from build123d import *

# Parameters (mm, degrees)
CHANFRO2_SIZE         = 0.3
CORTE_EXTRUS_O2_REACH = 10.374
ESBO_O7_W             = 0.5
ESBO_O7_H             = 0.2
PADR_OCIRCULAR1_COUNT = 8
M2X0_4_TAPPED_HOLE1_D = 1.6


with BuildPart() as part:
    # Esboço2 → Revolução1 (revolve)
    with BuildSketch(Plane.XY, mode=Mode.PRIVATE) as revolu_o1_sk:
        Polygon((0, 8), (1.75, 8), (1.75, 5.7), (1.4, 5.7), (1.4, 2.3), (1.75, 2.3), (1.75, 0), (0, 0), align=None)
    revolve(revolu_o1_sk.sketch.rotate(Axis((0, 0, 0), (0, 1, 0)), 90), axis=Axis((0, 0, 0), (0, 1, 0)))

    # Chanfro2
    chanfro2_edges = [part.edges().sort_by_distance(p)[0] for p in [
        (0, 0, 1.75),
        (0, 8, 1.75),
    ]]
    chamfer(chanfro2_edges, length=CHANFRO2_SIZE)

    # Corte-extrusão2: up to this face of the body (flat: up to its plane)
    corte_extrus_o2_end = Plane(part.part.faces().sort_by_distance((0, 0, 0))[0])
    # Esboço7 → Corte-extrusão2 (cut, up to the picked face)
    with BuildSketch(Plane(origin=(0, 8, 0), x_dir=(1, 0, 0), z_dir=(0, 1, 0)), mode=Mode.PRIVATE) as corte_extrus_o2_sk1:
        with Locations((0, 1.65)):
            Rectangle(ESBO_O7_W, ESBO_O7_H)
    corte_extrus_o2_tool1 = split(extrude(corte_extrus_o2_sk1.sketch, amount=-CORTE_EXTRUS_O2_REACH, mode=Mode.PRIVATE), bisect_by=corte_extrus_o2_end, keep=Keep.BOTH, mode=Mode.PRIVATE)
    corte_extrus_o2 = corte_extrus_o2_tool1.solids().sort_by(Axis((0, 8, -1.65), (0, -1, 0)))[0]
    add(corte_extrus_o2, mode=Mode.SUBTRACT)

    # PadrãoCircular1: Corte-extrusão2 ×8 about axis
    padr_ocircular1_axis = Axis((0, 0, 0), (0, 1, 0))
    for i in range(1, PADR_OCIRCULAR1_COUNT):
        add(corte_extrus_o2.rotate(padr_ocircular1_axis, i * 360 / PADR_OCIRCULAR1_COUNT), mode=Mode.SUBTRACT)

    # M2x0.4 Tapped Hole1 (through all)
    with Locations(Plane(origin=(0, 8, 0), x_dir=(1, 0, 0), z_dir=(0, 1, 0))):
        with Locations((0, 0)):
            Hole(M2X0_4_TAPPED_HOLE1_D / 2)


solid = part.part
Read the model definition and answer for the solid it produces. Units are mm, in the model's axes. Round coordinates to 2 decimals unless told otherwise and drop trailing zeros. Write each loop counter-clockwise with the first axis right and the second up, starting at its lowest first coordinate (ties: lowest second). Pieces come first, ordered by that corner, then holes. Notation, with made-up numbers: (75, 29) - (124, 29) arc R15 ccw to (124, 40) - close; hole circle Ø6 at (36, 54.25). An arc over 180 degrees is marked (long way). One line per question, with ' | ' between items. Start each with the question number.
1. Section A-A (x = 0) is taken. Determine the outline of the cut face in (y, z).
2. Section D-D (y = 2.75) is taken. Determine the outline of the cut face in (x, z).
3. For a pull along Y with two mould halves and no side action, classify faces 1 (the face through (0.63, 3.94, 0.49)), 2 (the face through (-0.06, 3.98, 1.4)), 3 (the face through (0.6, 7.88, -1.45)) as +Y half, -Y half, draft (parallel to the pull), parting line (faces both ways), or undercut.
4. Find the intervals of material crossed by probe 1 along Z at (x, y) = (0.05, 3.25); probe 2 along Z at (x, y) = (0, 2); probe 3 along Z at (x, y) = (-1.45, 6.5), in increasing order. Write a range as [from, to].
5. Section B-B (z = 0) is taken. Determine the outline of the cut face in (x, y).
Filled in:
1) outline: (0, -1.45) - (0.1, -1.55) - (2.3, -1.55) - (2.3, -1.4) - (5.7, -1.4) - (5.7, -1.55) - (7.9, -1.55) - (8, -1.45) - (8, -0.8) - (0, -0.8) - close; (0, 0.8) - (8, 0.8) - (8, 1.45) - (7.9, 1.55) - (5.7, 1.55) - (5.7, 1.4) - (2.3, 1.4) - (2.3, 1.55) - (0.1, 1.55) - (0, 1.45) - close
2) outline: circle Ø2.8 at (0, 0); hole circle Ø1.6 at (0, 0)
3) face 1: draft | face 2: undercut | face 3: +Y half
4) probe 1: [-1.4, -0.8], [0.8, 1.4] | probe 2: [-1.55, -0.8], [0.8, 1.55] | probe 3: [-0.98, 0.98]
5) outline: (-1.55, 0.1) - (-1.45, 0) - (-0.8, 0) - (-0.8, 8) - (-1.45, 8) - (-1.55, 7.9) - (-1.55, 5.7) - (-1.4, 5.7) - (-1.4, 2.3) - (-1.55, 2.3) - close; (0.8, 0) - (1.45, 0) - (1.55, 0.1) - (1.55, 2.3) - (1.4, 2.3) - (1.4, 5.7) - (1.55, 5.7) - (1.55, 7.9) - (1.45, 8) - (0.8, 8) - close
